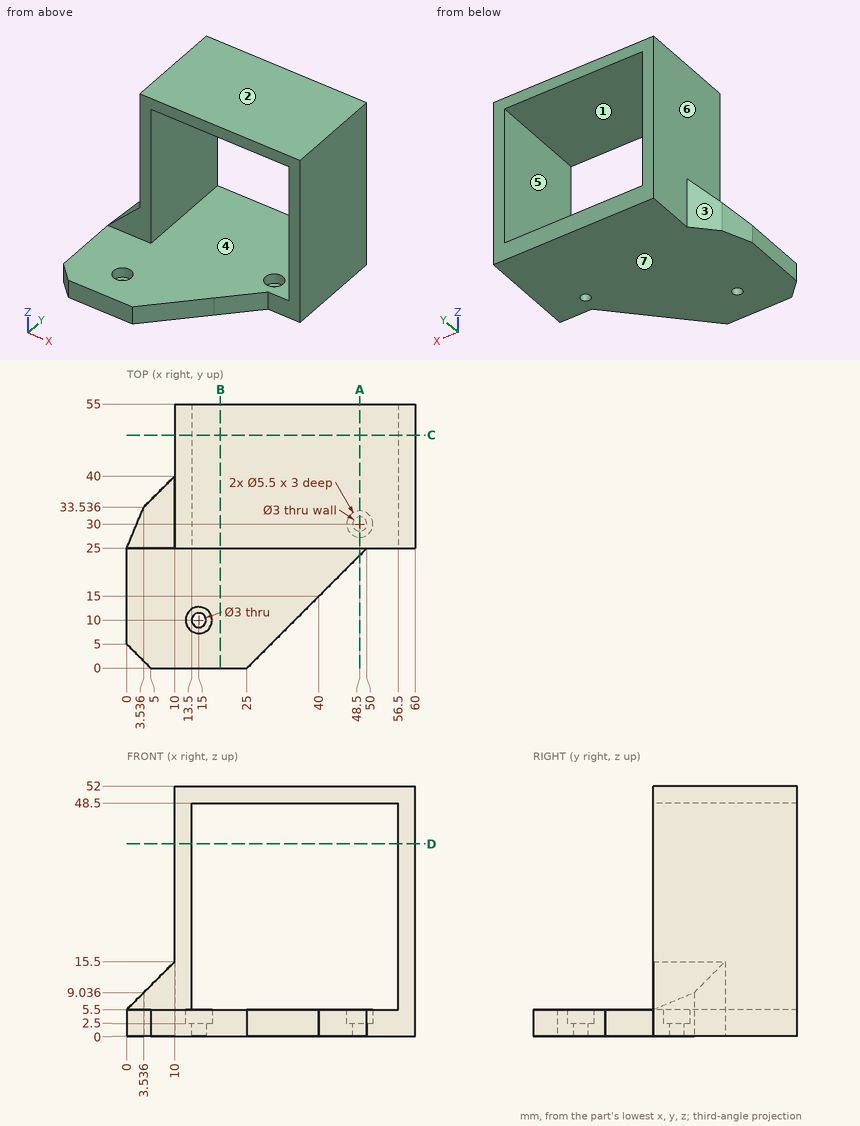
Source: three-view drawing plus pictorial views. Frame: mm from the lowest corner of the part. A direction names the side the tool comes from. Give positions to 0.01 mm unless a question says otherwise; leave off trailing zeros. Write each loop counter-clockwise with the first axis right and the second up, starting at its lowest first coordinate (ties: lowest second). Pieces come first, ordered by that corner, then holes. Notation, with made-up numbers: (16.25, 42.25) -> (61.25, 42.25) arc R35 cw to (61.25, 77.25) -> close; hole circle Ø11 at (12.25, 30). An arc over 180 degrees is marked (long way). Write item = value, one per line.
Q1. Cut plane A-A on x = 48.5. Return loops of the section in (y, z), then the cut area to 3 significant figures.
Here are the results:
outline = (23.5, 0) -> (28.5, 0) -> (28.5, 2.5) -> (27.25, 2.5) -> (27.25, 5.5) -> (23.5, 5.5) -> close; (25, 48.5) -> (55, 48.5) -> (55, 52) -> (25, 52) -> close; (31.5, 0) -> (55, 0) -> (55, 5.5) -> (32.75, 5.5) -> (32.75, 2.5) -> (31.5, 2.5) -> close
area = 254 mm²
Q2. Cut plane C-C on y = 48.5. Return loops of the section in (x, z), then the cut area to 3 significant figures.
Here are the results:
outline = (10, 0) -> (60, 0) -> (60, 52) -> (10, 52) -> close; hole (13.5, 5.5) -> (56.5, 5.5) -> (56.5, 48.5) -> (13.5, 48.5) -> close
area = 751 mm²
Q3. Cut plane D-D on z = 40. Return loops of the section in (x, y), then the cut area to 3 significant figures.
Here are the results:
outline = (10, 25) -> (13.5, 25) -> (13.5, 55) -> (10, 55) -> close; (56.5, 25) -> (60, 25) -> (60, 55) -> (56.5, 55) -> close
area = 210 mm²
Q4. Line query: line 1 (Z direction, x = 25.5, y = 48); line 2 (X direction, y = 53, z = 43); line 3 (Z direction, x = 44.5, y = 22). Output: solid intervals per line, ascending. Write a range as from..to.
Here are the results:
line_1 = 0..5.5, 48.5..52
line_2 = 10..13.5, 56.5..60
line_3 = 0..5.5
Q5. Mould query, pull axis Z, two halves, no side actions, for the marked faces 1, 2 and 3. Classes: +Z half, -Z half, draft (parallel to the pull), parting line (faces both ways), or undercut.
Here are the results:
face_1 = undercut
face_2 = +Z half
face_3 = draft
Q6. Reachability of the marked faces 4, 5, 6 and 7 from +Z, -Z, +X, -X, +Y, -Y: full face, straight path, thin tool, end or side. Return the list, or none.
Here are the results:
face_4 = -Y
face_5 = +Y, -Y
face_6 = +Z, -X, +Y
face_7 = -Z, +X, -X, +Y, -Y
Q7. Cut plane B-B on x = 19.5. Return loops of the section in (y, z).
Here are the results:
outline = (0, 0) -> (55, 0) -> (55, 5.5) -> (0, 5.5) -> close; (25, 48.5) -> (55, 48.5) -> (55, 52) -> (25, 52) -> close
Q8. First-contact query: pin 1 (9 mm diameter, centred on y = 42.5, z = 19.5, fed in from -X); pin 2 (12 mm diameter, centred on x = 30, z = 46, fed in from -Y); pin 3 (4.5 mm diameter, centred on x = 16, y = 11.5, fed in from +Z); pin 4 (8 mm diameter, centred on y = 18, z = 46.5, fed in from +X). Flat tips, straight axial feed; report the tip coordinate or a pass-through.
Here are the results:
pin_1 = 10
pin_2 = 25
pin_3 = 5.5
pin_4 = through
